Build history of the part. All positions in model axes, mm. Face numbers are marked on the shaded views. A direction names the side the tool comes from. Round coordinates to 2 decimals unless told otherwise and drop trailing zeros. Write each loop counter-clockwise with the first axis right and the second up, starting at its lowest first coordinate (ties: lowest second). Pieces come first, ordered by that corner, then holes.
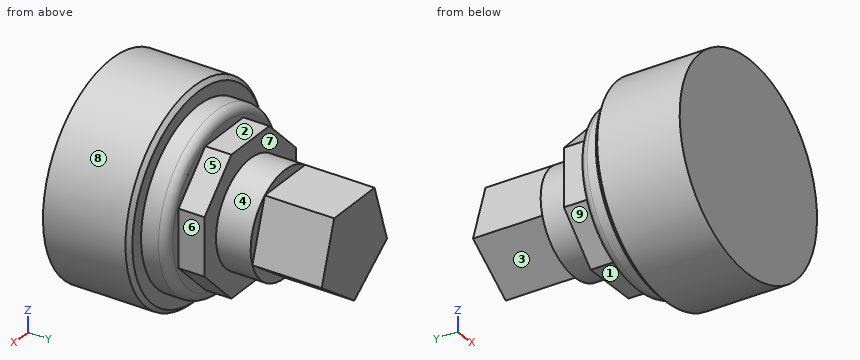
from build123d import *

# Parameters (mm, degrees)
SKETCH2_R           = 38.1
BOSS_EXTRUDE1_DEPTH = 31.75
CHAMFER1_SIZE       = 1.524
SKETCH3_R           = 31.75
BOSS_EXTRUDE3_DEPTH = 9.525
FILLET1_R           = 3.175
BOSS_EXTRUDE4_DEPTH = 9.525
SKETCH5_R           = 19.05
BOSS_EXTRUDE5_DEPTH = 12.7
BOSS_EXTRUDE6_DEPTH = 25.4


with BuildPart() as part:
    # Sketch2 → Boss-Extrude1 (new body)
    with BuildSketch(Plane(origin=(0, 0, 0), x_dir=(1, 0, 0), z_dir=(0, 1, 0))):
        with Locations(Location((0, 0, 0), (0, 0, 270))):
            Circle(SKETCH2_R)
    extrude(amount=BOSS_EXTRUDE1_DEPTH)

    # Chamfer1
    chamfer1_edges = [part.edges().sort_by_distance(p)[0] for p in [
        (0, 31.75, -38.1),
    ]]
    chamfer(chamfer1_edges, length=CHAMFER1_SIZE)

    # Sketch3 → Boss-Extrude3 (add)
    with BuildSketch(Plane(origin=(0, 31.75, 0), x_dir=(1, 0, 0), z_dir=(0, 1, 0))):
        with Locations(Location((0, 0, 0), (0, 0, 90))):
            Circle(SKETCH3_R)
    extrude(amount=BOSS_EXTRUDE3_DEPTH)

    # Fillet1
    fillet1_edges = [part.edges().sort_by_distance(p)[0] for p in [
        (0, 41.275, 31.75),
    ]]
    fillet(fillet1_edges, radius=FILLET1_R)

    # Sketch4 → Boss-Extrude4 (add)
    with BuildSketch(Plane(origin=(0, 41.275, 0), x_dir=(1, 0, 0), z_dir=(0, 1, 0))):
        Polygon((25.4, 10.521024484), (10.521024484, 25.4), (-10.521024484, 25.4), (-25.4, 10.521024484), (-25.4, -10.521024484), (-10.521024484, -25.4), (10.521024484, -25.4), (25.4, -10.521024484), align=None)
    extrude(amount=BOSS_EXTRUDE4_DEPTH)

    # Sketch5 → Boss-Extrude5 (add)
    with BuildSketch(Plane(origin=(0, 50.8, 0), x_dir=(1, 0, 0), z_dir=(0, 1, 0))):
        with Locations(Location((0, 0, 0), (0, 0, 270))):
            Circle(SKETCH5_R)
    extrude(amount=BOSS_EXTRUDE5_DEPTH)

    # Sketch6 → Boss-Extrude6 (add)
    with BuildSketch(Plane(origin=(0, 63.5, 0), x_dir=(1, 0, 0), z_dir=(0, 1, 0))):
        Polygon((-11.197309056, -15.411773743), (11.197309056, -15.411773743), (18.117626635, 5.886773743), (0, 19.05), (-18.117626635, 5.886773743), align=None)
    extrude(amount=BOSS_EXTRUDE6_DEPTH)


solid = part.part
1) Mould opens along X. For the marked faces 6, 7, 8 and 9 say: released by +X, released by -X, zero draft, split by the parting line, or undercut.
Results:
face 6: released by +X
face 7: zero draft
face 8: split by the parting line
face 9: released by -X
2) Wall check: L1, parallel to Y at x = -30, z = -11.5; L2, parallel to Z at x = -5, y = 44; L3, parallel to Y at x = 21, z = 10.5. Give the ranges that are in metal, low to high.
Results:
L1: y = 0 to 31.75
L2: z = -25.4 to 25.4
L3: y = 0 to 50.8
3) Pin check, flat tips, straight feed: pin 1 Ø6 at (y, z) = (26.5, -30.5) entering from -X; pin 2 Ø7.5 at (x, y) = (3.5, 47.5) entering from -Z; pin 3 Ø12 at (y, z) = (60.5, 9.5) entering from +X. Stop position of each tip, or through.
Results:
pin 1: stops at x = -26.37
pin 2: stops at z = -25.4
pin 3: stops at x = 18.73
4) Slice it at A-A (y = 11). Write the cut outline in (x, z), plus the area to 3 significant figures.
Results:
outline: circle Ø76.2 at (0, 0)
area: 4,560 mm2
5) Which spindle directions (+Z, -Z, +X, -X, +Y, -Y) get a long thin tool onto all of the face, cutting with end or side? Do the marked faces 1, 2, 3, 4 and 5. Say none if no direction does.
Results:
face 1: -Z, +X, -X, +Y
face 2: +Z, +X, -X, +Y
face 3: -Z, -X, +Y
face 4: +Y
face 5: +Z, +X, +Y
6) Slice it at B-B (z = 0). Write the cut outline in (x, y) (3 decimals), plus the area to 3 significant figures.
Results:
outline: (-38.1, 0) - (38.1, 0) - (38.1, 30.226) - (36.576, 31.75) - (31.75, 31.75) - (31.75, 38.1) arc R3.175 ccw to (28.575, 41.275) - (25.4, 41.275) - (25.4, 50.8) - (19.05, 50.8) - (19.05, 63.5) - (16.205, 63.5) - (16.205, 88.9) - (-16.205, 88.9) - (-16.205, 63.5) - (-19.05, 63.5) - (-19.05, 50.8) - (-25.4, 50.8) - (-25.4, 41.275) - (-28.575, 41.275) arc R3.175 ccw to (-31.75, 38.1) - (-31.75, 31.75) - (-36.576, 31.75) - (-38.1, 30.226) - close
area: 4,810 mm2
7) Slice it at C-C (y = 35.5). Write the cut outline in (x, z).
Results:
outline: circle Ø63.5 at (0, 0)
